Geometry: final body of the model. Coordinates: model frame, mm. Face numbers are marked on the shaded views. A direction names the side the tool comes from. Round coordinates to 2 decimals unless told otherwise and drop trailing zeros. Loops run counter-clockwise (first coordinate to the right, second up) from the corner with the lowest first, then second, coordinate; pieces in that order, holes last. Notation, with made-up numbers: (67.25, -2.75) - (87.25, -2.75) arc R20 ccw to (87.25, 22.25) - close; hole circle Ø11 at (10.5, 56). An arc over 180 degrees is marked (long way). Use CSV: the item, a comma, the result in double quotes.
from build123d import *

# Parameters (mm, degrees)
ESQUISSE1_W             = 15.04863884
ESQUISSE1_H             = 8.025940715
BOSS_EXTRU_2_DEPTH      = 15
ESQUISSE2_R             = 1.5
ENL_V_MAT_EXTRU_1_DEPTH = 22
ESQUISSE7_R             = 1.5
ENL_V_MAT_EXTRU_2_DEPTH = 22
ESQUISSE8_R             = 5
ESQUISSE8_R_2           = 1.5
BOSS_EXTRU_3_DEPTH      = 40


with BuildPart() as part:
    # Esquisse1 → Boss.-Extru.2 (new body)
    with BuildSketch(Plane.XY):
        with BuildLine():
            Line((-20.404811956, 60.852158428), (-20.404811956, 43.608028339))
            Line((-20.404811956, 43.608028339), (-140.404811956, 43.608028339))
            ThreePointArc((-140.404811956, 43.608028339), (-170.122450923, 30.625328971), (-180.789117416, 0))
            ThreePointArc((-180.789117416, 0), (-170.122450923, -30.625328971), (-140.404811956, -43.608028339))
            Line((-140.404811956, -43.608028339), (-20.404811956, -43.608028339))
            Line((-20.404811956, -43.608028339), (-20.404811956, -60.852158428))
            Line((-20.404811956, -60.852158428), (-20.404811956, -80))
            Line((-20.404811956, -80), (0, -80))
            Line((0, -80), (0, 80))
            Line((0, 80), (-20.404811956, 80))
            Line((-20.404811956, 80), (-20.404811956, 60.852158428))
        make_face()
        with Locations((-50.437129359, 24.595057981)):
            Rectangle(ESQUISSE1_W, ESQUISSE1_H, mode=Mode.SUBTRACT)
        with Locations((-50.437129359, -24.595057981)):
            Rectangle(ESQUISSE1_W, ESQUISSE1_H, mode=Mode.SUBTRACT)
    extrude(amount=BOSS_EXTRU_2_DEPTH)

    # Esquisse2 → Enlèv. mat.-Extru.1 (cut)
    with BuildSketch(Plane(origin=(-170.122450923, 30.625328971, 0), x_dir=(0, 0, 1), z_dir=(-0.7337061397658711, 0.6794669237496878, 0))):
        with Locations(Location((3.566685756, 8.282361033, 0), (0, 0, 270))):
            Circle(ESQUISSE2_R)
        with Locations(Location((3.566685756, -21.717638967, 0), (0, 0, 270))):
            Circle(ESQUISSE2_R)
        with Locations(Location((3.566685756, -6.717638967, 0), (0, 0, 270))):
            Circle(ESQUISSE2_R)
    extrude(amount=-ENL_V_MAT_EXTRU_1_DEPTH, mode=Mode.SUBTRACT)

    # Esquisse7 → Enlèv. mat.-Extru.2 (cut)
    with BuildSketch(Plane(origin=(-170.122450923, -30.625328971, 15), x_dir=(0, 0, 1), z_dir=(-0.7337061397658707, -0.6794669237496883, 0))):
        with Locations(Location((-11.555586861, 21.717638967, 0), (0, 0, 270))):
            Circle(ESQUISSE7_R)
        with Locations(Location((-11.555586861, -8.282361033, 0), (0, 0, 270))):
            Circle(ESQUISSE7_R)
        with Locations(Location((-11.555586861, 6.717638967, 0), (0, 0, 270))):
            Circle(ESQUISSE7_R)
    extrude(amount=-ENL_V_MAT_EXTRU_2_DEPTH, mode=Mode.SUBTRACT)

    # Esquisse8 → Boss.-Extru.3 (add)
    # profile 1 of 6: a face of its own
    with BuildSketch(Plane.XY.offset(15)):
        with Locations(Location((-9.890580264, 72.213588888, 0), (0, 0, 180))):
            Circle(ESQUISSE8_R)
        with Locations((-9.890580264, 72.213588888)):
            Circle(ESQUISSE8_R_2, mode=Mode.SUBTRACT)
    # profile 2 of 6: a face of its own
    with BuildSketch(Plane.XY.offset(15)):
        with Locations(Location((-9.890580264, -71.991912234, 0), (0, 0, 180))):
            Circle(ESQUISSE8_R)
        with Locations((-9.890580264, -71.991912234)):
            Circle(ESQUISSE8_R_2, mode=Mode.SUBTRACT)
    # profile 3 of 6: a face of its own
    with BuildSketch(Plane.XY.offset(15)):
        with Locations(Location((-27.465625713, 36.162213608, 0), (0, 0, 180))):
            Circle(ESQUISSE8_R)
        with Locations((-27.465625713, 36.162213608)):
            Circle(ESQUISSE8_R_2, mode=Mode.SUBTRACT)
    # profile 4 of 6: a face of its own
    with BuildSketch(Plane.XY.offset(15)):
        with Locations(Location((-29.042873382, -37.067142431, 0), (0, 0, 180))):
            Circle(ESQUISSE8_R)
        with Locations((-29.042873382, -37.067142431)):
            Circle(ESQUISSE8_R_2, mode=Mode.SUBTRACT)
    # profile 5 of 6: a face of its own
    with BuildSketch(Plane.XY.offset(15)):
        with Locations(Location((-144.181953183, 36.162213608, 0), (0, 0, 180))):
            Circle(ESQUISSE8_R)
        with Locations((-144.181953183, 36.162213608)):
            Circle(ESQUISSE8_R_2, mode=Mode.SUBTRACT)
    # profile 6 of 6: a face of its own
    with BuildSketch(Plane.XY.offset(15)):
        with Locations(Location((-144.181953183, -37.067142431, 0), (0, 0, 180))):
            Circle(ESQUISSE8_R)
        with Locations((-144.181953183, -37.067142431)):
            Circle(ESQUISSE8_R_2, mode=Mode.SUBTRACT)
    extrude(amount=BOSS_EXTRU_3_DEPTH)


solid = part.part
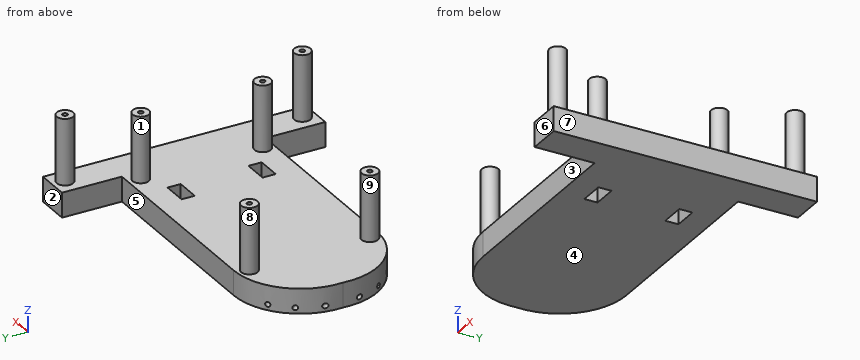
Item 1: Material intervals for line 1 (Y direction, x = -56.5, z = 11); line 2 (Z direction, x = -28, y = -37); line 3 (X direction, y = 34.5, z = 31), sorted ascending.
Final values:
line 1,"y = -43.61 to -28.61, -20.58 to 20.58, 28.61 to 43.61"
line 2,"z = 0 to 15"
line 3,"x = -148.9 to -139.47, -32.18 to -22.75"
Item 2: Pin query (flat end, axial travel): P1, Ø1.5, axis at x = -144, y = 36.5, coming from the +Z side; P2, Ø16.5, axis at y = -60.5, z = 10.5, coming from the -X side; P3, Ø12, axis at x = -106, z = 6.5, coming from the -Y side. Return the tip coordinate at first contact, or that it passes through.
Final values:
P1,"stops at z = 15"
P2,"stops at x = -20.4"
P3,"stops at y = -43.61"
Item 3: Section A-A on z = 33. Give the number of separate pieces and of enclosed holes in the cut face, plus the area to 3 significant figures.
Final values:
separate pieces,"6"
enclosed holes,"6"
area,"429 mm²"
Item 4: Reachability of the marked faces 1, 2, 3, 4 and 5 from +Z, -Z, +X, -X, +Y, -Y: full face, straight path, thin tool, end or side. Return the list, or none.
Final values:
face 1,"+Z"
face 2,"+Z, -Z, +X, -X, +Y"
face 3,"+Z, -Z, -X, -Y"
face 4,"-Z, +X, -X, +Y, -Y"
face 5,"+Z, -Z, -X, +Y"
Item 5: Mould query, pull axis Y, two halves, no side actions, for the marked faces 6, 7, 8 and 9. Classes: released by +Y, released by -Y, zero draft, split by the parting line, or undercut.
Final values:
face 6,"released by -Y"
face 7,"zero draft"
face 8,"undercut"
face 9,"undercut"
Item 6: Section B-B on x = -115.5. Return the cut outline in (y, z).
Final values:
outline,"(-43.61, 0) - (43.61, 0) - (43.61, 15) - (-43.61, 15) - close"
